Autodesk Inventor part; units mm, degrees
ref_plane "YZ Plane" through (0, 0, 0) normal (1, 0, 0) x (0, 1, 0)
ref_plane "XZ Plane" through (0, 0, 0) normal (0, 1, 0) x (-1, 0, 0)
ref_plane "XY Plane" through (0, 0, 0) normal (0, 0, 1) x (1, 0, 0)
sketch "Szkic1" plane through (0, 0, 0) normal (0, 1, 0) x (-1, 0, 0)
  circle A0 centre (0, 0) radius 6.5
  line L0 (1.7321, 3) -> (3.4641, 0)
  line L1 (3.4641, 0) -> (1.7321, -3)
  line L2 (1.7321, -3) -> (-1.7321, -3)
  line L3 (-1.7321, -3) -> (-3.4641, 0)
  line L4 (-3.4641, 0) -> (-1.7321, 3)
  line L5 (-1.7321, 3) -> (1.7321, 3)
  circle A1 centre (0, 0) radius 4
  dimension "d0" = 13
  dimension "d1" = 6
  dimension "d12" = 8
extrude "Wyciągnięcie proste1" add sketch "Szkic1" along normal blind 4 contours A0 | L0 L1 L2 L3 L4 L5 | A1
extrude "Wyciągnięcie proste2" add sketch "Szkic1" against normal blind 4 contours A0 | A1
sketch "Szkic2" plane through (0, 4, 0) normal (0, 1, 0) x (1, 0, 0)
  circle A0 centre (0, 0) radius 4
  dimension "d7" = 8
extrude "Wyciągnięcie proste3" add sketch "Szkic2" along normal blind 90
thread "Gwint1"
thread "Gwint2"
properties part number "M8x80_threaded"
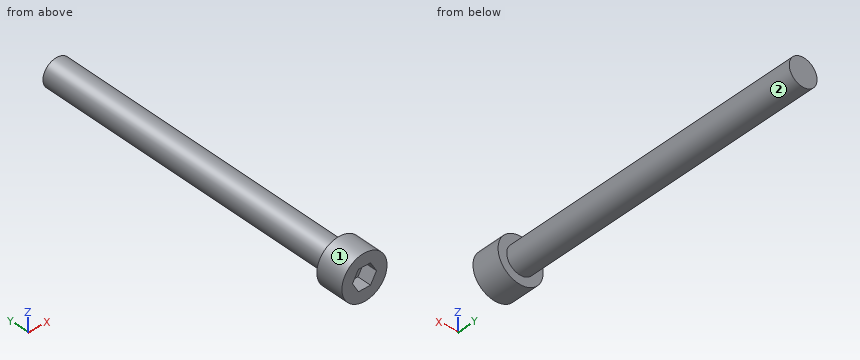
Work out the finished part from the listing and answer in its coordinate system (mm). Face numbers are marked on the shaded views. A direction names the side the tool comes from. Give positions to 0.01 mm unless a question says otherwise; leave off trailing zeros. Order: outer loops, then holes, each group sorted by start corner. A loop starts at its lowest first (then second) coordinate and runs counter-clockwise, first axis right, second up. Notation, with made-up numbers: (40.5, -23) -> (98.5, -23) arc R28 ccw to (98.5, 7) -> close; hole circle Ø11 at (36.5, 80.5). An arc over 180 degrees is marked (long way). One line per item, written item: value.
Item 1: A tool of negligible diameter and unlimited length cuts with its end or side. For the marked faces 1 and 2, from which of +Z, -Z, +X, -X, +Y, -Y can it reach the whole face along a straight path? Write none if from no direction.
Answer sheet:
face 1: +Y, -Y
face 2: +Y
Item 2: Find section B-B, the plane z = 1.75. Give the vertices of the cut face in (x, y).
Answer sheet:
outline: (-6.26, -4) -> (-2.45, -4) -> (-2.45, 0) -> (2.45, 0) -> (2.45, -4) -> (6.26, -4) -> (6.26, 4) -> (3.6, 4) -> (3.6, 94) -> (-3.6, 94) -> (-3.6, 4) -> (-6.26, 4) -> close
Item 3: Straight lines are drawn through the part: probe 1 along Y at (x, z) = (-0.5, 0.5); probe 2 along Y at (x, z) = (-3.5, 4.75). For each, find the intervals that lie inside material, in ascending order.
Answer sheet:
probe 1: 0 to 94
probe 2: -4 to 4
Item 4: Find section C-C, the plane y = 59. Give the vertices of the cut face in (x, z).
Answer sheet:
outline: circle Ø8 at (0, 0)
Item 5: Find section D-D, the plane z = -5.25. Give the vertices of the cut face in (x, y), plus the area to 3 significant figures.
Answer sheet:
outline: (-3.83, -4) -> (3.83, -4) -> (3.83, 4) -> (-3.83, 4) -> close
area: 61.3 mm²
Item 6: Find section A-A, the plane x = 0. Give the vertices of the cut face in (y, z).
Answer sheet:
outline: (-4, -6.5) -> (4, -6.5) -> (4, -4) -> (94, -4) -> (94, 4) -> (4, 4) -> (4, 6.5) -> (-4, 6.5) -> (-4, 3) -> (0, 3) -> (0, -3) -> (-4, -3) -> close
Item 7: Flat-ended cylindrical pins translate along their axes: P1, Ø1.7, axis at x = 0.5, y = -2, coming from the +Z side; P2, Ø3, axis at x = 0, z = -1, coming from the -Y side; P3, Ø1.5, axis at x = 3, y = 12, coming from the +Z side; P4, Ø2, axis at x = -4, y = 62.5, coming from the -Z side. Find the tip coordinate at first contact, or state that the pin passes through.
Answer sheet:
P1: z = 6.5
P2: y = 0
P3: z = 3.31
P4: z = -2.65
